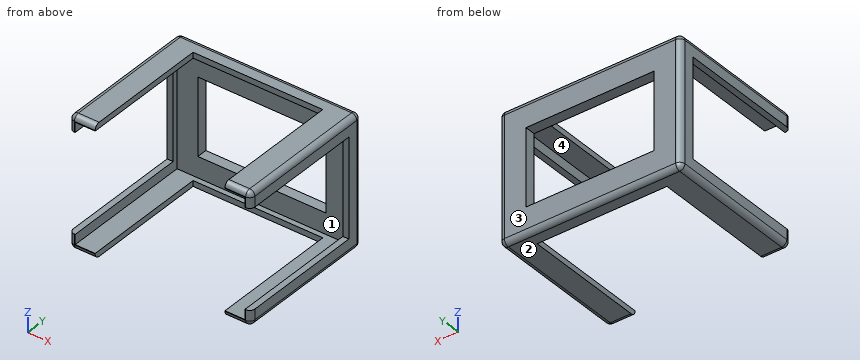
```python
from build123d import *

# Parameters (mm, degrees)
SKETCH1_W               = 88.9
SKETCH1_H               = 63.5
BOSS_EXTRUDE2_DEPTH     = 69.85
FILLET2_R               = 2.54
CUT_EXTRUDE1_START      = -5.08
SKETCH3_W               = 83.058
SKETCH3_H               = 57.912
CUT_EXTRUDE1_DEPTH      = 65.77
SKETCH5_W               = 63.5
SKETCH5_H               = 76.2
CUT_EXTRUDE3_DEPTH      = 1
CUT_EXTRUDE3_DEPTH_BACK = 64.5
SKETCH6_W               = 48.26
SKETCH6_H               = 76.2
CUT_EXTRUDE4_DEPTH      = 1
CUT_EXTRUDE4_DEPTH_BACK = 89.9
SKETCH7_W               = 62.738
SKETCH7_H               = 37.592
CUT_EXTRUDE5_DEPTH      = 6.08


with BuildPart() as part:
    # Sketch1 → Boss-Extrude2 (new body)
    with BuildSketch(Plane(origin=(0, 0, 0), x_dir=(1, 0, 0), z_dir=(0, 1, 0))):
        with Locations((44.45, -31.75)):
            Rectangle(SKETCH1_W, SKETCH1_H)
    extrude(amount=BOSS_EXTRUDE2_DEPTH)

    # Fillet2
    fillet2_edges = [part.edges().sort_by_distance(p)[0] for p in [
        (88.9, 69.85, 31.75),
        (44.45, 69.85, 0),
        (0, 69.85, 31.75),
        (44.45, 0, 0),
        (88.9, 0, 31.75),
        (44.45, 0, 63.5),
        (0, 0, 31.75),
        (0, 34.925, 0),
        (88.9, 34.925, 0),
        (88.9, 34.925, 63.5),
        (0, 34.925, 63.5),
        (44.45, 69.85, 63.5),
    ]]
    fillet(fillet2_edges, radius=FILLET2_R)

    # Sketch3 → Cut-Extrude1 (cut, through all)
    with BuildSketch(Plane(origin=(0, 69.85, 0), x_dir=(1, 0, 0), z_dir=(0, 1, 0)).offset(CUT_EXTRUDE1_START)):
        with Locations((44.45, -31.75)):
            Rectangle(SKETCH3_W, SKETCH3_H)
    extrude(amount=-CUT_EXTRUDE1_DEPTH, mode=Mode.SUBTRACT)

    # Sketch5 → Cut-Extrude3 (cut, two sides)
    with BuildSketch(Plane.XY.offset(63.5)) as cut_extrude3_sk:
        with Locations((44.45, 24.13)):
            Rectangle(SKETCH5_W, SKETCH5_H)
    extrude(amount=CUT_EXTRUDE3_DEPTH, mode=Mode.SUBTRACT)
    extrude(cut_extrude3_sk.sketch, amount=-CUT_EXTRUDE3_DEPTH_BACK, mode=Mode.SUBTRACT)

    # Sketch6 → Cut-Extrude4 (cut, two sides)
    with BuildSketch(Plane.ZY) as cut_extrude4_sk:
        with Locations((31.75, 24.13)):
            Rectangle(SKETCH6_W, SKETCH6_H)
    extrude(amount=CUT_EXTRUDE4_DEPTH, mode=Mode.SUBTRACT)
    extrude(cut_extrude4_sk.sketch, amount=-CUT_EXTRUDE4_DEPTH_BACK, mode=Mode.SUBTRACT)

    # Sketch7 → Cut-Extrude5 (cut, through all)
    with BuildSketch(Plane.XZ.offset(-64.77)):
        with Locations((44.45, 31.75)):
            Rectangle(SKETCH7_W, SKETCH7_H)
    extrude(amount=-CUT_EXTRUDE5_DEPTH, mode=Mode.SUBTRACT)


solid = part.part
```
Read the model definition and answer for the solid it produces. Units are mm, in the model's axes. Face numbers are marked on the shaded views. A direction names the side the tool comes from. Give positions to 0.01 mm unless a question says otherwise; leave off trailing zeros. Order: outer loops, then holes, each group sorted by start corner. A loop starts at its lowest first (then second) coordinate and runs counter-clockwise, first axis right, second up. Notation, with made-up numbers: (89.25, 55.5) -> (117.25, 55.5) arc R12 ccw to (117.25, 76.5) -> close; hole circle Ø11 at (-8.5, 14). An arc over 180 degrees is marked (long way). One line per item, written item: value. Start each with the question number.
(1) The part is cut by section A-A (z = 31). Determine the outline of the cut face in (x, y), and give its area (3 significant figures).
(2) The part is cut by section D-D (z = 52). Determine the outline of the cut face in (x, y), and give its area (3 significant figures).
(3) Flat-ended cylindrical pins translate along their axes: P1, Ø3, axis at x = 87.5, z = 20.5, coming from the -Y side; P2, Ø2, axis at y = 34, z = 62.5, coming from the +X side; P3, Ø1.5, axis at x = 1, y = 26.5, coming from the -Z side. Find the tip coordinate at first contact, or state that the pin passes through.
(4) The part is cut by section C-C (x = 65). Determine the outline of the cut face in (y, z), and give its area (3 significant figures).
(5) Straight lines are drawn through the part: L1, parallel to X at y = 30, z = 58; L2, parallel to X at y = 66.5, z = 38; L3, parallel to Z at x = 51.5, y = 64.5. For each, find the intervals that lie inside material, in ascending order.
(6) A tool of negligible diameter and unlimited length cuts with its end or side. For the marked faces 3 and 4, from which of +Z, -Z, +X, -X, +Y, -Y can it reach the whole face along a straight path? Write none if from no direction.
(7) The part is cut by section B-B (y = 21). Determine the outline of the cut face in (x, z).
(8) For a pull along X with two mould halves and no side action, classify the marked faces 1 and 2 as released by +X, released by -X, zero draft, split by the parting line, or undercut.
Taken from the geometry:
1. outline: (0, 62.23) -> (2.92, 62.23) -> (2.92, 64.77) -> (13.08, 64.77) -> (13.08, 69.85) -> (2.54, 69.85) arc R2.54 ccw to (0, 67.31) -> close; (75.82, 64.77) -> (85.98, 64.77) -> (85.98, 62.23) -> (88.9, 62.23) -> (88.9, 67.31) arc R2.54 ccw to (86.36, 69.85) -> (75.82, 69.85) -> close
1. area: 145 mm^2
2. outline: (0, 62.23) -> (2.92, 62.23) -> (2.92, 64.77) -> (85.98, 64.77) -> (85.98, 62.23) -> (88.9, 62.23) -> (88.9, 67.31) arc R2.54 ccw to (86.36, 69.85) -> (2.54, 69.85) arc R2.54 ccw to (0, 67.31) -> close
2. area: 464 mm^2
3. P1: y = 62.23
3. P2: x = 88.84
3. P3: z = 0.13
4. outline: (62.23, 0) -> (67.31, 0) arc R2.54 ccw to (69.85, 2.54) -> (69.85, 12.95) -> (64.77, 12.95) -> (64.77, 2.79) -> (62.23, 2.79) -> close; (62.23, 60.71) -> (64.77, 60.71) -> (64.77, 50.55) -> (69.85, 50.55) -> (69.85, 60.96) arc R2.54 ccw to (67.31, 63.5) -> (62.23, 63.5) -> close
4. area: 143 mm^2
5. L1: 0 to 2.92, 85.98 to 88.9
5. L2: 0 to 13.08, 75.82 to 88.9
5. L3: 0 to 2.79, 60.71 to 63.5
6. face 3: +Z, -Z, +X, -X, +Y
6. face 4: -Y
7. outline: (0, 2.54) arc R2.54 ccw to (2.54, 0) -> (12.7, 0) -> (12.7, 2.79) -> (2.92, 2.79) -> (2.92, 7.62) -> (0, 7.62) -> close; (0, 55.88) -> (2.92, 55.88) -> (2.92, 60.71) -> (12.7, 60.71) -> (12.7, 63.5) -> (2.54, 63.5) arc R2.54 ccw to (0, 60.96) -> close; (76.2, 0) -> (86.36, 0) arc R2.54 ccw to (88.9, 2.54) -> (88.9, 7.62) -> (85.98, 7.62) -> (85.98, 2.79) -> (76.2, 2.79) -> close; (76.2, 60.71) -> (85.98, 60.71) -> (85.98, 55.88) -> (88.9, 55.88) -> (88.9, 60.96) arc R2.54 ccw to (86.36, 63.5) -> (76.2, 63.5) -> close
8. face 1: undercut
8. face 2: zero draft
